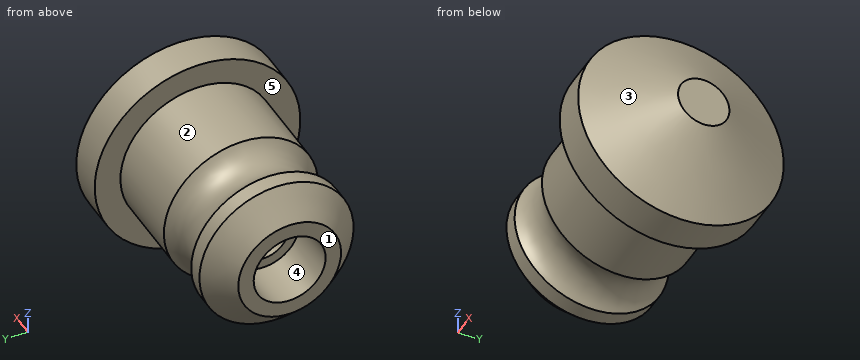
from build123d import *


with BuildPart() as f1:
    # F0 (on Front) → F1 (revolve)
    with BuildSketch(Plane.XZ):
        with BuildLine():
            Line((-26.660254, 0), (-1, 0))
            Line((-1, 0), (-1, 5))
            Line((-1, 5), (-9.660254, 20))
            Line((-9.660254, 20), (-16.660254, 20))
            Line((-16.660254, 20), (-16.660254, 15))
            Line((-16.660254, 15), (-33.168647, 15))
            ThreePointArc((-33.168647, 15), (-38.360685, 12.40621), (-43.552724, 15))
            Line((-43.552724, 15), (-46.660254, 15))
            Line((-46.660254, 15), (-51.660254, 10))
            Line((-51.660254, 10), (-51.660254, 7))
            Line((-51.660254, 7), (-41.660254, 7))
            Line((-41.660254, 7), (-41.660254, 5))
            Line((-41.660254, 5), (-26.660254, 5))
            Line((-26.660254, 5), (-26.660254, 0))
        make_face()
    revolve(axis=Axis((-30.367628, 0, 0), (1, 0, 0)))


solid = f1.part
The model under review builds one solid part; all positions refer to its coordinate system, in mm. Face numbers are marked on the shaded views. A direction names the side the tool comes from. Give positions to 0.01 mm unless a question says otherwise; leave off trailing zeros. Loops run counter-clockwise (first coordinate to the right, second up) from the corner with the lowest first, then second, coordinate; pieces in that order, holes last. Notation, with made-up numbers: (74.5, 71) -> (86.5, 71) arc R14 ccw to (86.5, 84) -> close; hole circle Ø1 at (-16.75, -11). An arc over 180 degrees is marked (long way). Answer as a JSON object with one key per item and string values. Group by question number.
Q1. Wall thickness on line 1 along Z through (x, y) = (-30, 0); line 2 along Z through (x, y) = (-45, 0): over which ranges is each line inside the solid? List them lowest first.
Q2. Take a section at C-C (x = -30.5). Write out the cut boundary in (y, z), plus the area to 3 significant figures.
Q3. Insertion check: pin 1 (4 mm diameter, centred on x = -11, y = -13.5, fed in from -Z); pin 2 (7 mm diameter, centred on y = 2, z = 2.5, fed in from -X); pin 3 (2 mm diameter, centred on x = -11.5, y = -4.5, fed in from -Z). Each pin has a flat end and moves straight along its axis. Give the tip position at first contact, or say it passes through.
Q4. Take a section at A-A (y = 0). Write out the cut boundary in (x, z), plus the area to 3 significant figures.
Q5. Draft analysis for pull direction Z (two halves, no side actions). For the marked faces 3, 4 and 5, state which applies: pulls with the +Z half, pulls with the -Z half, needs draft (parallel to the pull), parting line crosses it, or undercut.
Q6. Tool access review of the marked faces 1 and 2: name each direction out of +Z, -Z, +X, -X, +Y, -Y from which nothing blocks a thin tool from reaching the whole face with its end or side.
Answer below:
{
 "1": {"line 1": "z = -15 to -5, 5 to 15", "line 2": "z = -15 to -7, 7 to 15"},
 "2": {"outline": "circle Ø30 at (0, 0); hole circle Ø10 at (0, 0)", "area": "628 mm2"},
 "3": {"pin 1": "stops at z = -16.36", "pin 2": "stops at x = -41.66", "pin 3": "stops at z = -19.69"},
 "4": {"outline": "(-51.66, -10) -> (-46.66, -15) -> (-43.55, -15) arc R6.49 cw to (-33.17, -15) -> (-16.66, -15) -> (-16.66, -20) -> (-9.66, -20) -> (-1, -5) -> (-1, 5) -> (-9.66, 20) -> (-16.66, 20) -> (-16.66, 15) -> (-33.17, 15) arc R6.49 cw to (-43.55, 15) -> (-46.66, 15) -> (-51.66, 10) -> (-51.66, 7) -> (-41.66, 7) -> (-41.66, 5) -> (-26.66, 5) -> (-26.66, -5) -> (-41.66, -5) -> (-41.66, -7) -> (-51.66, -7) -> close", "area": "1,190 mm2"},
 "5": {"face 3": "parting line crosses it", "face 4": "undercut", "face 5": "needs draft"},
 "6": {"face 1": "+Z, -Z, -X, +Y, -Y", "face 2": "-X"}
}
